Design review of the part built by this model. Coordinates are the model's own, in mm. A direction names the side the tool comes from. Coordinates: 2 decimals unless noted, no trailing zeros. Write each loop counter-clockwise with the first axis right and the second up, starting at its lowest first coordinate (ties: lowest second). Pieces come first, ordered by that corner, then holes.
Q1. Take a section at D-D, the plane z = 4.75. Write out the cut boundary in (x, y).
Q2. Take a section at A-A, the plane z = 1. Write out the cut boundary in (x, y).
Q3. For pin 1 Ø0.6 at (x, z) = (7.5, -1.5) entering from -Y; pin 2 Ø0.7 at (x, y) = (0, -7.5) entering from +Z; pin 3 Ø0.8 at (x, y) = (3.5, 2.5) entering from +Z, all flat-tipped, find the tip position at first contact; note any pin that passes through.
Q4. Take a section at C-C, the plane x = 6.25. Write out the cut boundary in (y, z), plus the area to 3 significant figures.
Q5. Take a section at B-B, the plane y = 2. Write out the cut boundary in (x, z), plus the area to 3 significant figures.
Q6. For L1, parallel to X at y = 1, z = 2.5; L2, parallel to Z at x = 4.25, y = 1.5; L3, parallel to Z at x = 6.25, y = -7.5, list the stretches that pass through material, from the lowest coordinate up.
Q7. The part is to be moulded in two halves that separate along X. For faces 1 (the flat face through (4, 2, 4.5)), 2 (the flat face through (4, -4, 5.5)), say which applies: released by +X, released by -X, zero draft, split by the parting line, or undercut.
Q8. For faces 3 (the flat face through (4, 3.04, 3)), 4 (the flat face through (3.06, 2, 5)), list the 3-axis set-ups (+Z, -Z, +X, -X, +Y, -Y) from which the entire face can be reached by the end or side of a thin tool; tool diameter is ignored.
from build123d import *

# Parameters (mm, degrees)
PAD002_DEPTH = 0.3
PAD_DEPTH    = 6.85
POCKET_DEPTH = 1
PAD001_DEPTH = 0.3


with BuildPart() as pad002:
    # Sketch002 → Pad002 (new body, symmetric)
    with BuildSketch(Plane.XZ.offset(7.62)):
        Polygon((-0.2, -3), (0.2, -3), (0.2, 2.12), (7.42, 2.12), (7.42, -3), (7.82, -3), (7.82, 2.52), (-0.2, 2.52), align=None)
    extrude(amount=PAD002_DEPTH, both=True)


with BuildPart() as pocket:
    # Sketch → Pad (new body, symmetric)
    with BuildSketch(Plane.XZ.offset(3.81)):
        Polygon((1.01, 0.2), (6.61, 0.2), (7.11, 2.32), (6.61, 5.5), (1.01, 5.5), (0.51, 2.32), align=None)
    extrude(amount=PAD_DEPTH, both=True)

    # Sketch003 → Pocket (cut)
    with BuildSketch(Plane(origin=(0, -3.81, 5.5), x_dir=(-1, 0, 0), z_dir=(0, 0, 1))):
        with BuildLine():
            ThreePointArc((-3.06, -5.35), (-3.81, -4.6), (-4.56, -5.35))
            Line((-4.56, -5.35), (-4.56, -6.85))
            Line((-4.56, -6.85), (-3.06, -6.85))
            Line((-3.06, -6.85), (-3.06, -5.35))
        make_face()
    extrude(amount=-POCKET_DEPTH, mode=Mode.SUBTRACT)


with BuildPart() as obj1:
    # Sketch001 → Pad001 (new body, symmetric)
    with BuildSketch(Plane.XZ):
        Polygon((-0.2, -3), (0.2, -3), (0.2, 2.12), (7.42, 2.12), (7.42, -3), (7.82, -3), (7.82, 2.52), (-0.2, 2.52), align=None)
    extrude(amount=PAD001_DEPTH, both=True)

    add(pad002.part)
    add(pocket.part)


solid = obj1.part
Responses:
1. outline: (0.89, -10.66) - (6.73, -10.66) - (6.73, 3.04) - (4.56, 3.04) - (4.56, 1.54) arc R0.75 cw to (3.06, 1.54) - (3.06, 3.04) - (0.89, 3.04) - close
2. outline: (-0.2, -7.92) - (0.2, -7.92) - (0.2, -7.32) - (-0.2, -7.32) - close; (-0.2, -0.3) - (0.2, -0.3) - (0.2, 0.3) - (-0.2, 0.3) - close; (0.82, -10.66) - (6.8, -10.66) - (6.8, 3.04) - (0.82, 3.04) - close; (7.42, -7.92) - (7.82, -7.92) - (7.82, -7.32) - (7.42, -7.32) - close; (7.42, -0.3) - (7.82, -0.3) - (7.82, 0.3) - (7.42, 0.3) - close
3. pin 1: stops at y = -7.92
3. pin 2: stops at z = 2.52
3. pin 3: stops at z = 4.5
4. outline: (-10.66, 0.2) - (3.04, 0.2) - (3.04, 5.5) - (-10.66, 5.5) - close
4. area: 72.6 mm2
5. outline: (0.51, 2.32) - (1.01, 0.2) - (6.61, 0.2) - (7.11, 2.32) - (6.61, 5.5) - (4.56, 5.5) - (4.56, 4.5) - (3.06, 4.5) - (3.06, 5.5) - (1.01, 5.5) - close
5. area: 30.8 mm2
6. L1: x = 0.54 to 7.08
6. L2: z = 0.2 to 4.5
6. L3: z = 0.2 to 5.5
7. face 1: undercut
7. face 2: zero draft
8. face 3: +Z, -Z, +X, -X, +Y
8. face 4: +Z, +Y
